Build history of the part. All positions in model axes, mm. A direction names the side the tool comes from. Coordinates: 2 decimals unless noted, no trailing zeros. Order: outer loops, then holes, each group sorted by start corner. A loop starts at its lowest first (then second) coordinate and runs counter-clockwise, first axis right, second up. Notation, with made-up numbers: (-33.5, 13.5) - (18.5, 13.5) arc R30 ccw to (18.5, 35.5) - close; hole circle Ø5 at (79, -6). An arc over 180 degrees is marked (long way). Write each question's results on one line, items separated by ' | '.
Autodesk Inventor part; units mm, degrees
ref_plane "YZ Plane" through (0, 0, 0) normal (1, 0, 0) x (0, 1, 0)
ref_plane "XZ Plane" through (0, 0, 0) normal (0, 1, 0) x (-1, 0, 0)
ref_plane "XY Plane" through (0, 0, 0) normal (0, 0, 1) x (1, 0, 0)
sketch "Sketch1" plane through (0, 0, 0) normal (0, 1, 0) x (-1, 0, 0)
  line L0 (0, 5) -> (-12.44, 5)
  line L1 (-15.44, 2) -> (-15.44, -2)
  line L2 (-12.44, -5) -> (5, -5)
  line L3 (5, -5) -> (5, 0)
  arc A0 (-12.44, 5) -> (-15.44, 2) centre (-12.44, 2) ccw
  arc A1 (-15.44, -2) -> (-12.44, -5) centre (-12.44, -2) ccw
  arc A2 (5, 0) -> (0, 5) centre (0, 0) ccw
  point P0 (-15.44, -5)
  point P1 (-15.44, 5)
  dimension "d0" = 20.44
  dimension "d1" = 10
  dimension "d2" = 3
  dimension "d3" = 5
extrude "Extrusion1" add sketch "Sketch1" along normal blind 2.35
sketch "Sketch3" plane through (0, 0, 0) normal (0, -1, 0) x (1, 0, 0)
  arc A0 (5, 0) -> (-5, 0) centre (0, 0) ccw
  arc A1 (-5, -18) -> (5, -18) centre (0, -18) ccw
  line L0 (-5, 0) -> (-5, -5)
  line L1 (5, 0) -> (5, -5)
  arc A2 (-5, -18) -> (-5, -5) centre (-15, -11.5) ccw
  arc A3 (5, -5) -> (5, -18) centre (15, -11.5) ccw
  dimension "d6" = 5
  dimension "d7" = 18
  dimension "d8" = 5
  dimension "d9" = 5
  dimension "d11" = 15
  dimension "d12" = 15
extrude "Extrusion2" add sketch "Sketch3" against normal blind 6
sketch "Sketch4" plane through (0, 6, 0) normal (0, 1, 0) x (1, 0, 0)
  circle A0 centre (0, 0) radius 1.6
  dimension "d16" = 3.2
extrude "Extrusion3" cut sketch "Sketch4" against normal up to next
properties part number "glass clip" material "ABS Plastic"
1. Probe line 1 (Z direction, x = 0, y = 1.4); line 2 (X direction, y = 2.05, z = 0); line 3 (X direction, y = 4.2, z = 0). List the from-to ranges inside material, lowest first.
Solved:
line 1: z = -23 to -1.6, 1.6 to 5 | line 2: x = -5 to -1.6, 1.6 to 15.44 | line 3: x = -5 to -1.6, 1.6 to 5
2. Tool access for faces 1 (the face through (9, 1, -5)), 2 (the face through (-1.606, 3.625, 4.735)), 3 (the face through (5, 4, -2)), 4 (the face through (6, 1, 5)): list every direction of +Z, -Z, +X, -X, +Y, -Y with a clear straight run to the whole face (end or side of a thin tool).
Solved:
face 1: -Z, +X, +Y, -Y | face 2: +Z, +Y | face 3: +Z, -Z, +X, +Y | face 4: +Z, +X, -X, +Y, -Y
3. Drop flat-ended pins along their axis: pin 1 Ø1.2 at (x, y) = (10.5, 0.5) entering from -Z; pin 2 Ø12 at (x, z) = (5, -11.5) entering from -Y; pin 3 Ø3 at (y, z) = (4.5, -2) entering from +X; pin 4 Ø1.5 at (y, z) = (2.5, -16.5) entering from +X. Give the stop position or say it passes through.
Solved:
pin 1: stops at z = -5 | pin 2: stops at y = 0 | pin 3: stops at x = 5 | pin 4: stops at x = 4.55
4. Band-saw the part on D-D on y = 5.6. Give the cut face in (x, z).
Solved:
outline: (-5, -18) arc R5 ccw to (5, -18) arc R11.93 cw to (5, -5) - (5, 0) arc R5 ccw to (-5, 0) - (-5, -5) arc R11.93 cw to start; hole circle Ø3.2 at (0, 0)
5. Band-saw the part on A-A on y = 0.4. Give the cut face in (x, z).
Solved:
outline: (-5, -18) arc R5 ccw to (5, -18) arc R11.93 cw to (5, -5) - (12.44, -5) arc R3 ccw to (15.44, -2) - (15.44, 2) arc R3 ccw to (12.44, 5) - (0, 5) arc R5 ccw to (-5, 0) - (-5, -5) arc R11.93 cw to start; hole circle Ø3.2 at (0, 0)
6. Band-saw the part on C-C on z = -3.5. Give the cut face in (x, y).
Solved:
outline: (-5, 0) - (15.04, 0) - (15.04, 2.35) - (5, 2.35) - (5, 6) - (-5, 6) - close
